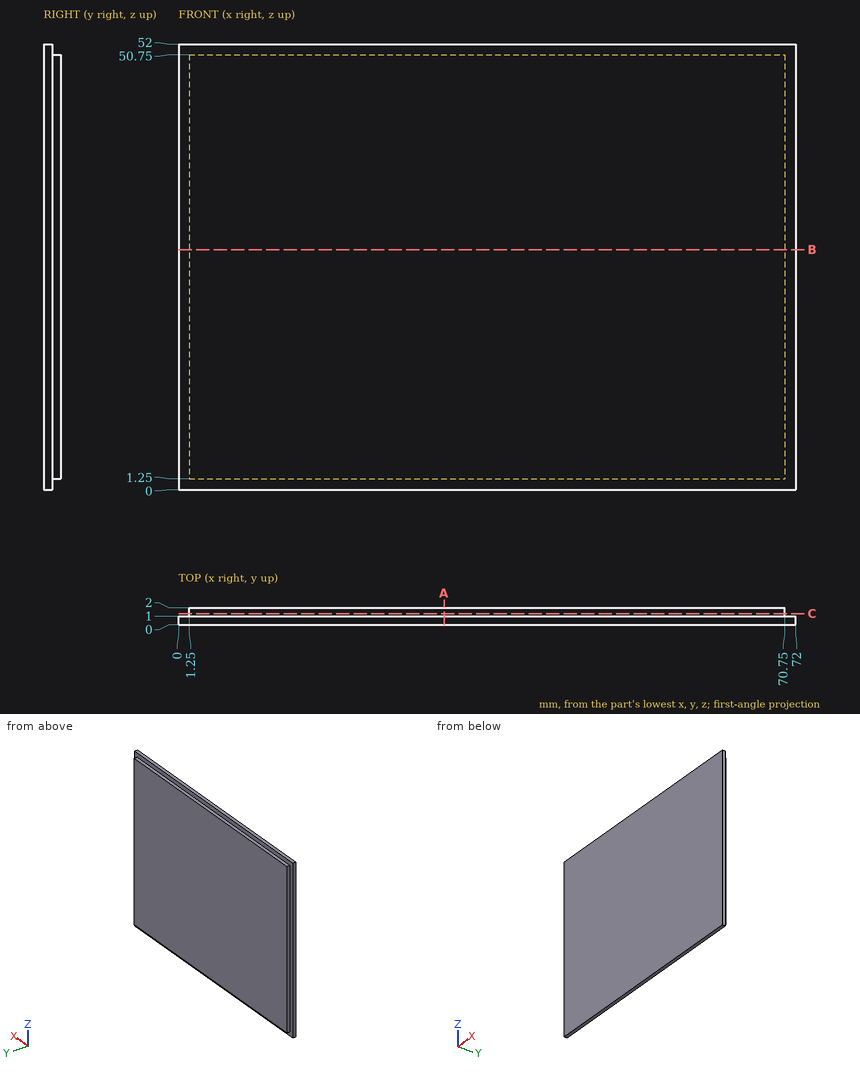
Answer from the drawing. Dimensions are ordinates in mm from the lowest x, y and z of the part. Round coordinates to 2 decimals unless told otherwise and drop trailing zeros. Write each loop counter-clockwise with the first axis right and the second up, starting at its lowest first coordinate (ties: lowest second). Pieces come first, ordered by that corner, then holes. Notation, with made-up numbers: M -8.75,6 L 20.25,6 A28 cw 20.25,35 Z; hole C 27.25,21 d1. An arc over 180 degrees is marked long. Write each question's results on one line, items separated by ' | '. Start each with the question number.
Item 1: Given pin 1 Ø0.8 at (y, z) = (1.5, 28.5) entering from -X; pin 2 Ø10 at (x, z) = (54, 32) entering from -Y; pin 3 Ø0.5 at (y, z) = (1.5, 19) entering from +X, each flat-ended and moving along its own axis, determine where each tip first touches the part or whether it passes through.
Item 2: Straight lines are drawn through the part: probe 1 along Z at (x, y) = (3, 1.25); probe 2 along X at (y, z) = (1.05, 47). For each, find the intervals that lie inside material, in ascending order.
Item 3: Find section C-C on y = 1.3. Write down the section's boundary in (x, z).
Item 4: Find section A-A on x = 31. Write down the section's boundary in (y, z), and give its area (4 significant figures).
Item 5: Find section B-B on z = 28. Write down the section's boundary in (x, y), and give its area (4 significant figures).
Answer block:
1) pin 1: stops at x = 1.25 | pin 2: stops at y = 0 | pin 3: stops at x = 70.75
2) probe 1: z = 1.25 to 50.75 | probe 2: x = 1.25 to 70.75
3) outline: M 1.25,1.25 L 70.75,1.25 L 70.75,50.75 L 1.25,50.75 Z
4) outline: M 0,0 L 1,0 L 1,1.25 L 2,1.25 L 2,50.75 L 1,50.75 L 1,52 L 0,52 Z | area: 101.5 mm²
5) outline: M 0,0 L 72,0 L 72,1 L 70.75,1 L 70.75,2 L 1.25,2 L 1.25,1 L 0,1 Z | area: 141.5 mm²
